from build123d import *

# Parameters (mm, degrees)
SALIENTE_EXTRUIR1_DEPTH = 3
REDONDEO1_R             = 10
CROQUIS2_R              = 1.5
CROQUIS2_R_2            = 2.05
CROQUIS2_W              = 42
CROQUIS2_H              = 20
CORTAR_EXTRUIR1_DEPTH   = 135.610141171
CROQUIS3_W              = 4
CROQUIS3_H              = 14.636342218
CORTAR_EXTRUIR2_DEPTH   = 135.610141171
CROQUIS4_W              = 44
CROQUIS4_H              = 22
CORTAR_EXTRUIR3_DEPTH   = 131.820067673


with BuildPart() as part:
    # Croquis1 → Saliente-Extruir1 (new body)
    with BuildSketch(Plane(origin=(0, 0, 0), x_dir=(1, 0, 0), z_dir=(0, 1, 0))):
        Polygon((-88.1, 42.318171109), (88.1, 42.318171109), (108.1, 22.318171109), (127.75, 22.318171109), (127.75, 7.681828891), (105.75, 7.681828891), (77.75, -42.318171109), (-77.75, -42.318171109), (-105.75, 7.681828891), (-127.75, 7.681828891), (-127.75, 22.318171109), (-108.1, 22.318171109), align=None)
    extrude(amount=SALIENTE_EXTRUIR1_DEPTH)

    # Redondeo1
    redondeo1_edges = [part.edges().sort_by_distance(p)[0] for p in [
        (-88.1, 1.5, -42.318171109),
        (88.1, 1.5, -42.318171109),
        (108.1, 1.5, -22.318171109),
        (105.75, 1.5, -7.681828891),
        (77.75, 1.5, 42.318171109),
        (-77.75, 1.5, 42.318171109),
        (-105.75, 1.5, -7.681828891),
        (-108.1, 1.5, -22.318171109),
    ]]
    fillet(redondeo1_edges, radius=REDONDEO1_R)

    # Croquis2 → Cortar-Extruir1 (cut, through all)
    with BuildSketch(Plane(origin=(0, 3, 0), x_dir=(1, 0, 0), z_dir=(0, 1, 0))):
        with Locations(Location((70, -17.318171109, 0), (0, 0, 270))):
            Circle(CROQUIS2_R)
        with Locations(Location((-70, -17.318171109, 0), (0, 0, 270))):
            Circle(CROQUIS2_R)
        with Locations(Location((-119.996067812, 15, 0), (0, 0, 270))):
            Circle(CROQUIS2_R)
        with Locations(Location((119.996067812, 15, 0), (0, 0, 270))):
            Circle(CROQUIS2_R)
        with Locations(Location((-75, 32.318171109, 0), (0, 0, 270))):
            Circle(CROQUIS2_R)
        with Locations(Location((75, 32.318171109, 0), (0, 0, 270))):
            Circle(CROQUIS2_R)
        with Locations(Location((-11.5, -14.318171109, 0), (0, 0, 270))):
            Circle(CROQUIS2_R)
        with Locations(Location((11.5, -14.318171109, 0), (0, 0, 270))):
            Circle(CROQUIS2_R)
        with Locations(Location((-11.5, -37.318171109, 0), (0, 0, 270))):
            Circle(CROQUIS2_R)
        with Locations(Location((11.5, -37.318171109, 0), (0, 0, 270))):
            Circle(CROQUIS2_R)
        with Locations(Location((-61, 7.318171109, 0), (0, 0, 270))):
            Circle(CROQUIS2_R_2)
        with Locations(Location((-11, 7.318171109, 0), (0, 0, 270))):
            Circle(CROQUIS2_R_2)
        with Locations(Location((-61, 13.318171109, 0), (0, 0, 270))):
            Circle(CROQUIS2_R_2)
        with Locations(Location((-61, 1.318171109, 0), (0, 0, 270))):
            Circle(CROQUIS2_R_2)
        with Locations(Location((-11, 13.318171109, 0), (0, 0, 270))):
            Circle(CROQUIS2_R_2)
        with Locations(Location((-11, 1.318171109, 0), (0, 0, 270))):
            Circle(CROQUIS2_R_2)
        with Locations((-36, 7.318171109)):
            Rectangle(CROQUIS2_W, CROQUIS2_H)
    extrude(amount=-CORTAR_EXTRUIR1_DEPTH, mode=Mode.SUBTRACT)

    # Croquis3 → Cortar-Extruir2 (cut, through all)
    with BuildSketch(Plane(origin=(0, 3, 0), x_dir=(1, 0, 0), z_dir=(0, 1, 0))):
        with Locations((-125.75, 15)):
            Rectangle(CROQUIS3_W, CROQUIS3_H)
        with Locations((125.75, 15)):
            Rectangle(CROQUIS3_W, CROQUIS3_H)
    extrude(amount=-CORTAR_EXTRUIR2_DEPTH, mode=Mode.SUBTRACT)

    # Croquis4 → Cortar-Extruir3 (cut, through all)
    with BuildSketch(Plane(origin=(0, 3, 0), x_dir=(1, 0, 0), z_dir=(0, 1, 0))):
        with Locations((-36, 7.318171109)):
            Rectangle(CROQUIS4_W, CROQUIS4_H)
    extrude(amount=-CORTAR_EXTRUIR3_DEPTH, mode=Mode.SUBTRACT)


solid = part.part
The listing builds one solid part. Answer for the finished solid, in the listing's coordinates (mm). Round coordinates to 2 decimals unless told otherwise and drop trailing zeros. Order: outer loops, then holes, each group sorted by start corner. A loop starts at its lowest first (then second) coordinate and runs counter-clockwise, first axis right, second up. Notation, with made-up numbers: M -15.5,60 L 4.5,60 A19 ccw 4.5,84 Z; hole C 24,-25 d5. An arc over 180 degrees is marked long. Answer in a Markdown table with one row per item. Add a question column.
1) Flat-ended cylindrical pins translate along their axes: pin 1 Ø2.5 at (x, z) = (-11, -13.32) entering from +Y; pin 2 Ø1 at (y, z) = (2.5, 17) entering from -X; pin 3 Ø1 at (y, z) = (2.5, 18.5) entering from -X. Find the tip coordinate at first contact, or state that the pin passes through.
2) The part is cut by section A-A on x = 98. Determine the outline of the cut face in (y, z).
3) Determine the mould class of faces 1 (the face through (-98.2, 1.48, -32.22)), 2 (the face through (91.906, 1.479, 17.04)), 3 (the face through (2, 0, -1)), 4 (the face through (-58.97, 1.52, -1.59)) for opening direction Z: pulls with the +Z half, pulls with the -Z half, needs draft (parallel to the pull), parting line crosses it, or undercut.
4) The part is cut by section C-C on x = -100. Determine the outline of the cut face in (y, z).
5) The part is cut by section B-B on y = 1. Count the separate pieces of the cut face and the enclosed holes in it, plus the area to 3 significant figures.
6) Consider line 1 along Z through (x, y) = (-37, 2.65); line 2 along X through (y, z) = (1.8, -16); line 3 along X through (y, z) = (1.15, 14). Determine where each line is inside the solid, lowest interval first. Write a range as from..to.
Findings below:
| question | item | result |
|---|---|---|
| 1 | pin 1 | passes through |
| 1 | pin 2 | stops at x = -92.21 |
| 1 | pin 3 | stops at x = -91.37 |
| 2 | outline | M 0,-32.42 L 3,-32.42 L 3,6.16 L 0,6.16 Z |
| 3 | face 1 | pulls with the -Z half |
| 3 | face 2 | pulls with the +Z half |
| 3 | face 3 | needs draft |
| 3 | face 4 | undercut |
| 4 | outline | M 0,-30.42 L 3,-30.42 L 3,2.59 L 0,2.59 Z |
| 5 | separate pieces | 1 |
| 5 | enclosed holes | 17 |
| 5 | area | 15,600 mm² |
| 6 | line 1 | z = -42.32..-18.32, 3.68..42.32 |
| 6 | line 2 | x = -123.75..-121.11, -118.88..-58, -14..118.88, 121.11..123.75 |
| 6 | line 3 | x = -93.61..-12.97, -10.03..10.03, 12.97..93.61 |
